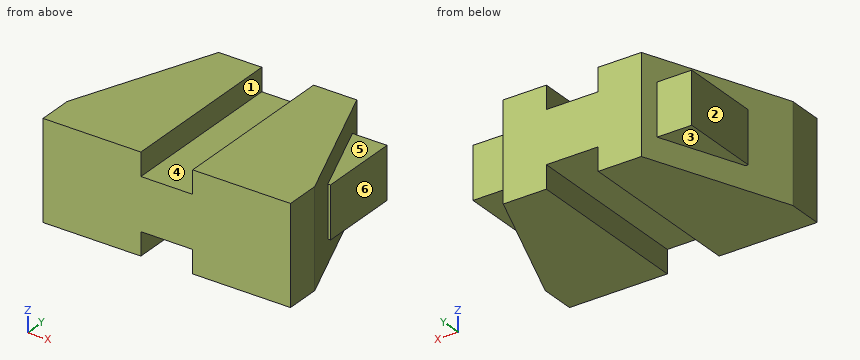
```python
from build123d import *

# Parameters (mm, degrees)
SKETCH1_W           = 86
SKETCH1_H           = 60
BOSS_EXTRUDE1_DEPTH = 17
SKETCH2_W           = 18
SKETCH2_H           = 8
CUT_EXTRUDE1_DEPTH  = 56.118055118
CUT_EXTRUDE3_DEPTH  = 56.118055118
SKETCH4_W           = 18
SKETCH4_H           = 28
BOSS_EXTRUDE2_DEPTH = 38


with BuildPart() as part:
    # Sketch1 → Boss-Extrude1 (new, symmetric)
    with BuildSketch(Plane.XY):
        Rectangle(SKETCH1_W, SKETCH1_H)
    extrude(amount=BOSS_EXTRUDE1_DEPTH, both=True)

    # Sketch2 → Cut-Extrude1 (cut, symmetric)
    with BuildSketch(Plane(origin=(0, 0, 0), x_dir=(1, 0, 0), z_dir=(0, 1, 0))):
        with Locations((0, -13)):
            Rectangle(SKETCH2_W, SKETCH2_H)
    cut_extrude1 = extrude(amount=CUT_EXTRUDE1_DEPTH, both=True, mode=Mode.SUBTRACT)

    # Mirror1: Cut-Extrude1 across plane
    add(cut_extrude1.mirror(Plane.XY), mode=Mode.SUBTRACT)

    # Sketch3 → Cut-Extrude3 (cut, symmetric)
    with BuildSketch(Plane.XY):
        Polygon((-43, 30), (-43, -18), (-24, 30), align=None)
    cut_extrude3 = extrude(amount=CUT_EXTRUDE3_DEPTH, both=True, mode=Mode.SUBTRACT)

    # Mirror2: Cut-Extrude3 across plane
    add(cut_extrude3.mirror(Plane(origin=(0, 0, 0), x_dir=(0, 0, 1), z_dir=(1, 0, 0))), mode=Mode.SUBTRACT)

    # Sketch4 → Boss-Extrude2 (add, symmetric)
    with BuildSketch(Plane(origin=(0, 0, 0), x_dir=(0, 0, -1), z_dir=(1, 0, 0))):
        with Locations((0, 11)):
            Rectangle(SKETCH4_W, SKETCH4_H)
    extrude(amount=BOSS_EXTRUDE2_DEPTH, both=True)


solid = part.part
```
Geometry: final body of the model. Coordinates: model frame, mm. Face numbers are marked on the shaded views. A direction names the side the tool comes from. Round coordinates to 2 decimals unless told otherwise and drop trailing zeros. Order: outer loops, then holes, each group sorted by start corner. A loop starts at its lowest first (then second) coordinate and runs counter-clockwise, first axis right, second up. Notation, with made-up numbers: (-36.5, 66) -> (-24.5, 66) arc R7 cw to (-24.5, 75) -> close; hole circle Ø6 at (61, 19). An arc over 180 degrees is marked (long way). Use one line per item in the form item = value. Start each with the question number.
1. Cut plane B-B (z = -3.5). Return the cut outline in (x, y).
2. Pin query (flat end, axial travel): pin 1 Ø9 at (y, z) = (17.5, -1.5) entering from -X; pin 2 Ø5 at (y, z) = (19.5, 4) entering from +X; pin 3 Ø3.5 at (x, y) = (-33.5, 13) entering from +Z. Return the tip coordinate at first contact, or that it passes through.
3. Reachability of the marked faces 1, 2 and 3 from +Z, -Z, +X, -X, +Y, -Y: full face, straight path, thin tool, end or side. Return the list, or none.
4. Draft query along X for the marked faces 4, 5 and 6. Return one class per face: pulls with the +X half, pulls with the -X half, needs draft (parallel to the pull), parting line crosses it, or undercut.
5. Cut plane A-A (z = -13). Return the cut outline in (x, y).
6. Cut plane D-D (x = 31). Return the cut outline in (y, z), then the cut area to 3 significant figures.
7. Cut plane C-C (y = -24). Return the cut outline in (x, z).
8. Line query: probe 1 along X at (y, z) = (-19, -11.5); probe 2 along Y at (x, z) = (-32, -5); probe 3 along Z at (x, y) = (-3, -21.5). Output: solid intervals per line, ascending.
Solution:
q1.outline = (-43, -30) -> (43, -30) -> (43, -18) -> (37.06, -3) -> (38, -3) -> (38, 25) -> (25.98, 25) -> (24, 30) -> (-24, 30) -> (-25.98, 25) -> (-38, 25) -> (-38, -3) -> (-37.06, -3) -> (-43, -18) -> close
q2.pin_1 = -38
q2.pin_2 = 38
q2.pin_3 = 9
q3.face_1 = +Z, +Y, -Y
q3.face_2 = +Z, -Z, -X, +Y
q3.face_3 = -Z, -X, +Y
q4.face_4 = undercut
q4.face_5 = needs draft
q4.face_6 = pulls with the +X half
q5.outline = (-43, -30) -> (-9, -30) -> (-9, 30) -> (-24, 30) -> (-43, -18) -> close; (9, -30) -> (43, -30) -> (43, -18) -> (24, 30) -> (9, 30) -> close
q6.outline = (-30, -17) -> (12.32, -17) -> (12.32, -9) -> (25, -9) -> (25, 9) -> (12.32, 9) -> (12.32, 17) -> (-30, 17) -> close
q6.area = 1,670 mm^2
q7.outline = (-43, -17) -> (-9, -17) -> (-9, -9) -> (9, -9) -> (9, -17) -> (43, -17) -> (43, 17) -> (9, 17) -> (9, 9) -> (-9, 9) -> (-9, 17) -> (-43, 17) -> close
q8.probe_1 = -43 to -9, 9 to 43
q8.probe_2 = -30 to 25
q8.probe_3 = -9 to 9
